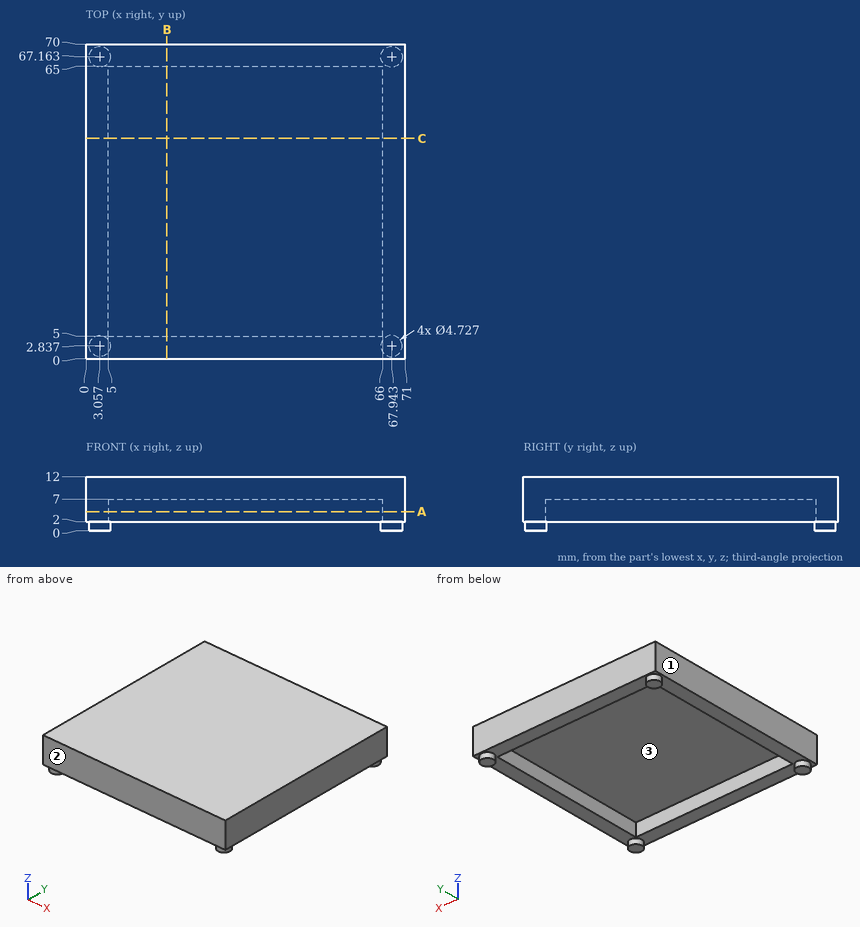
Geometry check sheet. Reference: drawing and pictorial views, mm from the part's lowest x, y, z. Give positions to 0.01 mm unless a question says otherwise; leave off trailing zeros. Order: outer loops, then holes, each group sorted by start corner. A loop starts at its lowest first (then second) coordinate and runs counter-clockwise, first axis right, second up.
1. Section check B-B, the plane x = 18. Enter the section's corners in (y, z).
2. Section check C-C, the plane y = 49. Enter the section's corners in (x, z), and give its area (3 significant figures).
3. Gauge pin test, flat end, axial feed: pin 1 Ø1 at (x, y) = (47, 44) entering from -Z. Record the tip position at first contact, or that the pin passes through.
4. Section check A-A, the plane z = 4.25. Enter the section's corners in (x, y), and give its area (3 significant figures).
5. Release check for a two-part mould opening along Y. For the marked faces 1, 2 and 3 record: pulls with the +Y half, pulls with the -Y half, needs draft (parallel to the pull), parting line crosses it, or undercut.
6. Thickness scan on L1, parallel to X at y = 12, z = 5.75; L2, parallel to Y at x = 13, z = 2.5; L3, parallel to Z at x = 55, y = 47. Record the ranges inside material, lowest first.
Values follow:
1. outline: (0, 2) - (5, 2) - (5, 7) - (65, 7) - (65, 2) - (70, 2) - (70, 12) - (0, 12) - close
2. outline: (0, 2) - (5, 2) - (5, 7) - (66, 7) - (66, 2) - (71, 2) - (71, 12) - (0, 12) - close
2. area: 405 mm2
3. pin 1: stops at z = 7
4. outline: (0, 0) - (71, 0) - (71, 70) - (0, 70) - close; hole (5, 5) - (66, 5) - (66, 65) - (5, 65) - close
4. area: 1,310 mm2
5. face 1: needs draft
5. face 2: pulls with the -Y half
5. face 3: undercut
6. L1: x = 0 to 5, 66 to 71
6. L2: y = 0 to 5, 65 to 70
6. L3: z = 7 to 12
